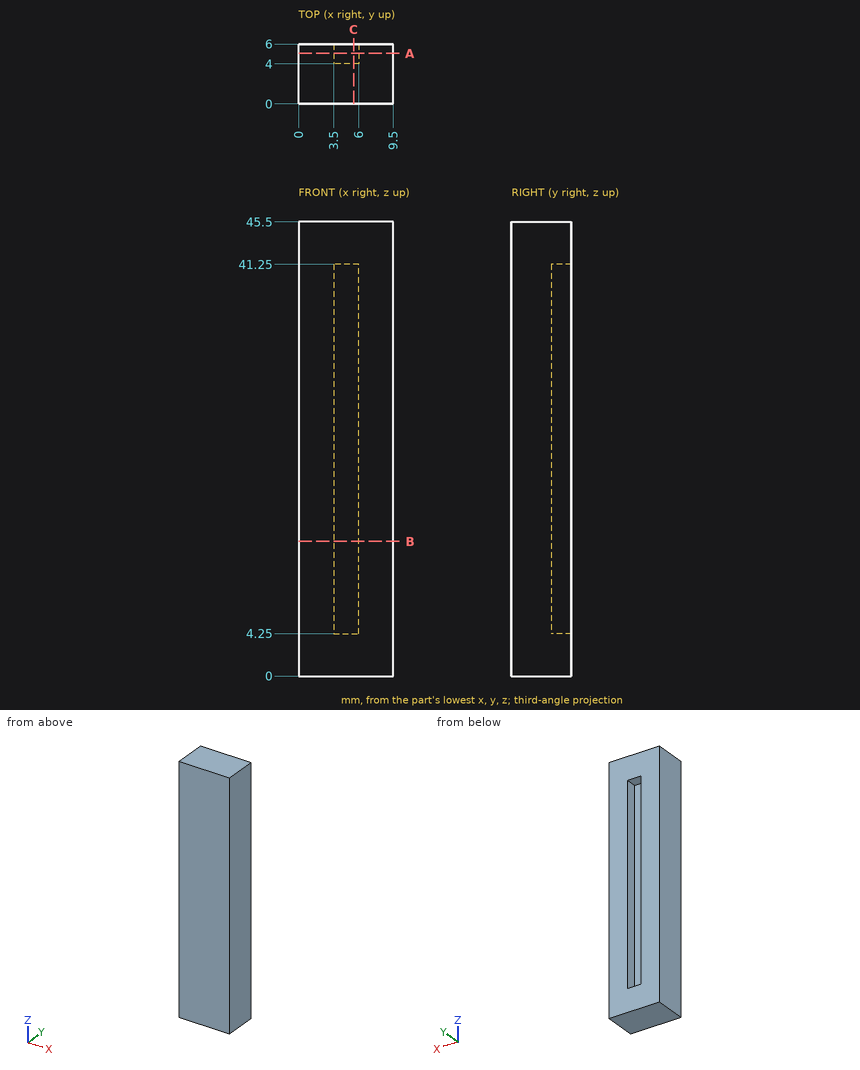
The figure shows three views and two pictorial views of one solid part (mm, origin at its lowest corner). Answer the questions. Give positions to 0.01 mm unless a question says otherwise; leave off trailing zeros. Order: outer loops, then holes, each group sorted by start corner. A loop starts at its lowest first (then second) coordinate and runs counter-clockwise, first axis right, second up. Notation, with made-up numbers: (-29, -33) - (10, -33) arc R16 ccw to (10, -2) - close; hole circle Ø5 at (87.5, 86.5). An arc over 180 degrees is marked (long way). Answer as CSV lines item,"result".
Q1. This flat-tipped pin is pushed along its axis until it touches: pin 1 Ø0.8 at (x, z) = (5, 29) entering from +Y. Where does it stop, or does it pass through?
Answer key:
pin 1,"stops at y = 4"
Q2. Straight lines are drawn through the part: L1, parallel to X at y = 5.2, z = 8; L2, parallel to Z at x = 5.25, y = 5.1; L3, parallel to Y at x = 4, z = 36. For each, find the intervals that lie inside material, in ascending order.
Answer key:
L1,"x = 0 to 3.5, 6 to 9.5"
L2,"z = 0 to 4.25, 41.25 to 45.5"
L3,"y = 0 to 4"
Q3. A cutting plane is placed at C-C, the plane x = 5.5. Determine the outline of the cut face in (y, z).
Answer key:
outline,"(0, 0) - (6, 0) - (6, 4.25) - (4, 4.25) - (4, 41.25) - (6, 41.25) - (6, 45.5) - (0, 45.5) - close"
Q4. A cutting plane is placed at A-A, the plane y = 5.05. Determine the outline of the cut face in (x, z).
Answer key:
outline,"(0, 0) - (9.5, 0) - (9.5, 45.5) - (0, 45.5) - close; hole (3.5, 4.25) - (6, 4.25) - (6, 41.25) - (3.5, 41.25) - close"
Q5. A cutting plane is placed at B-B, the plane z = 13.5. Determine the outline of the cut face in (x, y).
Answer key:
outline,"(0, 0) - (9.5, 0) - (9.5, 6) - (6, 6) - (6, 4) - (3.5, 4) - (3.5, 6) - (0, 6) - close"
